```python
from build123d import *

# Parameters (mm, degrees)
CYLINDER188_R          = 2
CYLINDER188_DEPTH      = 8
CYLINDER189_R          = 2
CYLINDER189_DEPTH      = 8
CYLINDER187_R          = 1.25
CYLINDER187_DEPTH      = 20
BOX018_W               = 3
BOX018_H               = 4
BOX018_DEPTH           = 5
BOX019_W               = 3
BOX019_H               = 4
BOX019_DEPTH           = 5
CYLINDER041_R          = 1.25
CYLINDER041_DEPTH      = 15
CYLINDER040_R          = 1.25
CYLINDER040_DEPTH      = 15
CYLINDER039_R          = 1.25
CYLINDER039_DEPTH      = 15
CYLINDER038_R          = 1.25
CYLINDER038_DEPTH      = 15
CYLINDER037_R          = 1.25
CYLINDER037_DEPTH      = 15
CYLINDER036_R          = 1.25
CYLINDER036_DEPTH      = 15
BOX015_W               = 10
BOX015_H               = 62
BOX015_DEPTH           = 32
BOX015_PLACEMENT_ANGLE = 3
BOX016_W               = 20
BOX016_H               = 10
BOX016_DEPTH           = 17
BOX017_W               = 10
BOX017_H               = 40
BOX017_DEPTH           = 17
BOX014_W               = 10
BOX014_H               = 62
BOX014_DEPTH           = 32
BOX014_PLACEMENT_ANGLE = 3
BOX013_W               = 20
BOX013_H               = 10
BOX013_DEPTH           = 17
CHAMFER_SIZE           = 5
CHAMFER001_SIZE        = 5
FILLET007_R            = 3
FILLET008_R            = 3


with BuildPart() as cylinder188:
    # Cylinder188 → Cylinder188 (new body)
    with BuildSketch(Plane(origin=(584, 7, 10.5), x_dir=(1, 0, 0), z_dir=(0, 0, 1))):
        Circle(CYLINDER188_R)
    extrude(amount=CYLINDER188_DEPTH)


with BuildPart() as fusion159:
    # Cylinder189 → Cylinder189 (new body)
    with BuildSketch(Plane(origin=(584, 55, 10.5), x_dir=(1, 0, 0), z_dir=(0, 0, 1))):
        Circle(CYLINDER189_R)
    extrude(amount=CYLINDER189_DEPTH)

    # Fusion159: union Cylinder188
    add(cylinder188.part)


with BuildPart() as fusion159_1:
    # Fusion159 placement: moved
    add(fusion159.part.moved(Location((0.5, 0, 0))))


with BuildPart() as cylinder187:
    # Cylinder187 → Cylinder187 (new body)
    with BuildSketch(Plane(origin=(586, 31, 1.5), x_dir=(1, 0, 0), z_dir=(0, 0, 1))):
        Circle(CYLINDER187_R)
    extrude(amount=CYLINDER187_DEPTH)


with BuildPart() as box018:
    # Box018 → Box018 (new body)
    with BuildSketch(Plane(origin=(580, 4, 1.5), x_dir=(1, 0, 0), z_dir=(0, 0, 1))):
        with Locations((1.5, 2)):
            Rectangle(BOX018_W, BOX018_H)
    extrude(amount=BOX018_DEPTH)


with BuildPart() as fusion032:
    # Box019 → Box019 (new body)
    with BuildSketch(Plane(origin=(580, 54, 1.5), x_dir=(1, 0, 0), z_dir=(0, 0, 1))):
        with Locations((1.5, 2)):
            Rectangle(BOX019_W, BOX019_H)
    extrude(amount=BOX019_DEPTH)

    # Fusion032: union Box018
    add(box018.part)


with BuildPart() as cylinder041:
    # Cylinder041 → Cylinder041 (new body)
    with BuildSketch(Plane(origin=(585, 7, 6), x_dir=(0, 0, -1), z_dir=(1, 0, 0))):
        Circle(CYLINDER041_R)
    extrude(amount=CYLINDER041_DEPTH)


with BuildPart() as fusion030:
    # Cylinder040 → Cylinder040 (new body)
    with BuildSketch(Plane(origin=(585, 7, 14), x_dir=(0, 0, -1), z_dir=(1, 0, 0))):
        Circle(CYLINDER040_R)
    extrude(amount=CYLINDER040_DEPTH)

    # Fusion030: union Cylinder041
    add(cylinder041.part)


with BuildPart() as fusion030_1:
    # Fusion030 placement: moved
    add(fusion030.part.moved(Location((0, 48, 0))))


with BuildPart() as cylinder039:
    # Cylinder039 → Cylinder039 (new body)
    with BuildSketch(Plane(origin=(585, 7, 6), x_dir=(0, 0, -1), z_dir=(1, 0, 0))):
        Circle(CYLINDER039_R)
    extrude(amount=CYLINDER039_DEPTH)


with BuildPart() as fusion031:
    # Cylinder038 → Cylinder038 (new body)
    with BuildSketch(Plane(origin=(585, 7, 14), x_dir=(0, 0, -1), z_dir=(1, 0, 0))):
        Circle(CYLINDER038_R)
    extrude(amount=CYLINDER038_DEPTH)

    # Fusion029: union Cylinder039
    add(cylinder039.part)

    # Fusion031: union Fusion030
    add(fusion030_1.part)


with BuildPart() as cylinder037:
    # Cylinder037 → Cylinder037 (new body)
    with BuildSketch(Plane(origin=(588, 61, 10), x_dir=(1, 0, 0), z_dir=(0, -1, 0))):
        Circle(CYLINDER037_R)
    extrude(amount=CYLINDER037_DEPTH)


with BuildPart() as fusion028:
    # Cylinder036 → Cylinder036 (new body)
    with BuildSketch(Plane(origin=(588, 16, 10), x_dir=(1, 0, 0), z_dir=(0, -1, 0))):
        Circle(CYLINDER036_R)
    extrude(amount=CYLINDER036_DEPTH)

    # Fusion028: union Cylinder037
    add(cylinder037.part)


with BuildPart() as box015:
    # Box015 → Box015 (new body)
    with BuildSketch(Plane.XY):
        with Locations((5, 31)):
            Rectangle(BOX015_W, BOX015_H)
    extrude(amount=BOX015_DEPTH)


with BuildPart() as box015_1:
    # Box015 placement: moved
    add(box015.part.moved(Location((600, 0, -3.6))).rotate(Axis((600, 0, -3.6), (0, -1, 0)), BOX015_PLACEMENT_ANGLE))


with BuildPart() as cut012:
    # Box016 → Box016 (new body)
    with BuildSketch(Plane(origin=(580, 0, 1.5), x_dir=(1, 0, 0), z_dir=(0, 0, 1))):
        with Locations((10, 5)):
            Rectangle(BOX016_W, BOX016_H)
    extrude(amount=BOX016_DEPTH)

    # Cut012: cut Box015
    add(box015_1.part, mode=Mode.SUBTRACT)


with BuildPart() as cut012_1:
    # Cut012 placement: moved
    add(cut012.part.moved(Location((0, 51, 0))))


with BuildPart() as box017:
    # Box017 → Box017 (new body)
    with BuildSketch(Plane(origin=(580, 11, 1.5), x_dir=(1, 0, 0), z_dir=(0, 0, 1))):
        with Locations((5, 20)):
            Rectangle(BOX017_W, BOX017_H)
    extrude(amount=BOX017_DEPTH)


with BuildPart() as box014:
    # Box014 → Box014 (new body)
    with BuildSketch(Plane.XY):
        with Locations((5, 31)):
            Rectangle(BOX014_W, BOX014_H)
    extrude(amount=BOX014_DEPTH)


with BuildPart() as box014_1:
    # Box014 placement: moved
    add(box014.part.moved(Location((600, 0, -3.6))).rotate(Axis((600, 0, -3.6), (0, -1, 0)), BOX014_PLACEMENT_ANGLE))


with BuildPart() as rear_cross_member:
    # Box013 → Box013 (new body)
    with BuildSketch(Plane(origin=(580, 0, 1.5), x_dir=(1, 0, 0), z_dir=(0, 0, 1))):
        with Locations((10, 5)):
            Rectangle(BOX013_W, BOX013_H)
    extrude(amount=BOX013_DEPTH)

    # Cut011: cut Box014
    add(box014_1.part, mode=Mode.SUBTRACT)


with BuildPart() as rear_cross_member_1:
    # Cut011 placement: moved
    add(rear_cross_member.part.moved(Location((0, 1, 0))))

    # Fusion022: union Cut012, Box017
    add(cut012_1.part)
    add(box017.part)

    # Chamfer
    chamfer_edges = [rear_cross_member_1.edges().sort_by_distance(p)[0] for p in [
        (590, 11, 10),
    ]]
    chamfer(chamfer_edges, length=CHAMFER_SIZE)

    # Chamfer001
    chamfer001_edges = [rear_cross_member_1.edges().sort_by_distance(p)[0] for p in [
        (590, 51, 10),
    ]]
    chamfer(chamfer001_edges, length=CHAMFER001_SIZE)

    # Fillet007
    fillet007_edges = [rear_cross_member_1.edges().sort_by_distance(p)[0] for p in [
        (589.86636, 61, 1.5),
        (589.420894, 61, 18.5),
    ]]
    fillet(fillet007_edges, radius=FILLET007_R)

    # Fillet008
    fillet008_edges = [rear_cross_member_1.edges().sort_by_distance(p)[0] for p in [
        (589.86636, 1, 1.5),
        (589.420894, 1, 18.5),
    ]]
    fillet(fillet008_edges, radius=FILLET008_R)

    # Cut015: cut Fusion028
    add(fusion028.part, mode=Mode.SUBTRACT)

    # Cut016: cut Fusion031
    add(fusion031.part, mode=Mode.SUBTRACT)

    # Cut017: cut Fusion032
    add(fusion032.part, mode=Mode.SUBTRACT)

    # Cut120: cut Cylinder187
    add(cylinder187.part, mode=Mode.SUBTRACT)

    # Cut121: cut Fusion159
    add(fusion159_1.part, mode=Mode.SUBTRACT)


solid = rear_cross_member_1.part
```
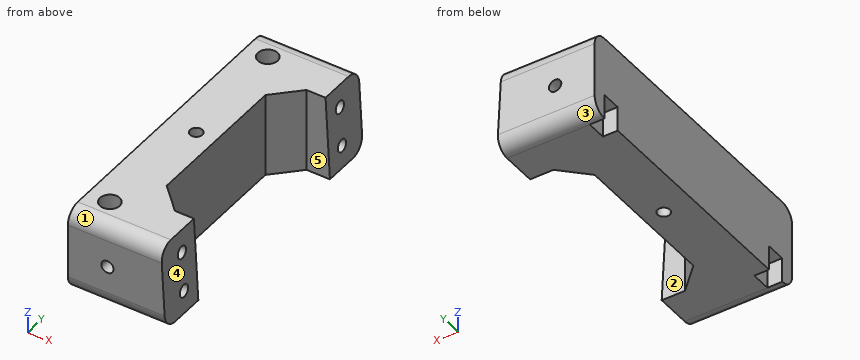
Input: part model. Units: mm. Frame: model coordinates. Face numbers are marked on the shaded views. A direction names the side the tool comes from. Coordinates: 2 decimals unless noted, no trailing zeros. Loops run counter-clockwise (first coordinate to the right, second up) from the corner with the lowest first, then second, coordinate; pieces in that order, holes last. Notation, with made-up numbers: M -26.75,46.5 L 29.25,46.5 A31 cw 29.25,83.5 Z; hole C 14,-27.5 d4. An arc over 180 degrees is marked long. Answer in a Markdown table with one row per item.
1. Reachability of the marked faces 1 and 2 from +Z, -Z, +X, -X, +Y, -Y: full face, straight path, thin tool, end or side. Return the list, or none.
Response:
| item | result |
|---|---|
| face 1 | +Z, +X, -X, -Y |
| face 2 | +Z, -Z, +X |
2. Section A-A, the plane x = 593.75. Output: boundary loops of the cut face in (y, z), then the cut area to 3 significant figures.
Response:
| item | result |
|---|---|
| outline | M 1,4.5 A3 ccw 4,1.5 L 12.25,1.5 L 12.25,18.5 L 4,18.5 A3 ccw 1,15.5 Z; M 49.75,1.5 L 58,1.5 A3 ccw 61,4.5 L 61,15.5 A3 ccw 58,18.5 L 49.75,18.5 Z; hole C 7,6 d2.5; hole C 7,14 d2.5; hole C 55,6 d2.5; hole C 55,14 d2.5 |
| area | 355 mm2 |
3. Draft query along Y for the marked faces 3, 4 and 5. Return one class per face: pulls with the +Y half, pulls with the -Y half, needs draft (parallel to the pull), parting line crosses it, or undercut.
Response:
| item | result |
|---|---|
| face 3 | pulls with the +Y half |
| face 4 | needs draft |
| face 5 | undercut |
4. First-contact query: pin 1 (2 mm diameter, centred on x = 588, z = 10, fed in from +Y); pin 2 (0.8 mm diameter, centred on x = 588, z = 10, fed in from -Y); pin 3 (1.5 mm diameter, centred on y = 55, z = 6, fed in from +X). Flat tips, straight axial feed; report the tip coordinate or a pass-through.
Response:
| item | result |
|---|---|
| pin 1 | stops at y = 46 |
| pin 2 | stops at y = 16 |
| pin 3 | stops at x = 585 |
5. Material intervals for line 1 (Z direction, x = 594.5, y = 7); line 2 (Y direction, x = 584.5, z = 12.5); line 3 (X direction, y = 31, z = 8.5), sorted ascending.
Response:
| item | result |
|---|---|
| line 1 | z = 1.5 to 4.75, 7.25 to 12.75, 15.25 to 18.5 |
| line 2 | y = 1 to 5, 9 to 53, 57 to 61 |
| line 3 | x = 580 to 584.75, 587.25 to 590 |
6. Section C-C, the plane y = 7. Output: boundary loops of the cut face in (x, z).
Response:
| item | result |
|---|---|
| outline | M 580,6.5 L 583,6.5 L 583,1.5 L 599.73,1.5 L 599.56,4.75 L 585,4.75 L 585,7.25 L 599.43,7.25 L 599.14,12.75 L 586.5,12.75 L 586.5,10.5 L 582.5,10.5 L 582.5,18.5 L 580,18.5 Z; M 586.5,15.25 L 599.01,15.25 L 598.84,18.5 L 586.5,18.5 Z; hole C 588,10 d2.5 |
7. Section B-B, the plane y = 31. Output: boundary loops of the cut face in (x, z).
Response:
| item | result |
|---|---|
| outline | M 580,1.5 L 584.75,1.5 L 584.75,18.5 L 580,18.5 Z; M 587.25,1.5 L 590,1.5 L 590,18.5 L 587.25,18.5 Z |
8. Section D-D, the plane z = 13.75. Output: boundary loops of the cut face in (x, y), then the cut area to 3 significant figures.
Response:
| item | result |
|---|---|
| outline | M 580,1 L 599.09,1 L 599.09,5.78 L 586.08,5.78 A2 cw long 586.08,8.22 L 599.09,8.22 L 599.09,11 L 595,11 L 590,16 L 590,46 L 595,51 L 599.09,51 L 599.09,53.78 L 586.08,53.78 A2 cw long 586.08,56.22 L 599.09,56.22 L 599.09,61 L 580,61 Z; hole C 586,31 d2.5 |
| area | 714 mm2 |
